Read the model definition and answer for the solid it produces. Units are mm, in the model's axes. Give positions to 0.01 mm unless a question says otherwise; leave off trailing zeros. Write each loop counter-clockwise with the first axis right and the second up, starting at its lowest first coordinate (ties: lowest second). Pieces come first, ordered by that corner, then holes. Notation, with made-up numbers: (50.25, 36) -> (66.25, 36) arc R26 cw to (66.25, 64) -> close; hole circle Ø5 at (-33, 80). An arc over 180 degrees is marked (long way). Write item = value, one per line.
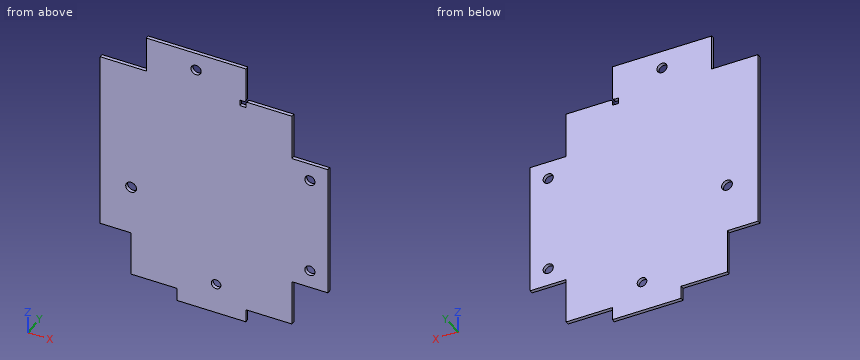
from build123d import *

# Parameters (mm, degrees)
CROQUIS1_W              = 190
CROQUIS1_H              = 230
SALIENTE_EXTRUIR2_DEPTH = 3
CROQUIS3_W              = 30
CROQUIS3_H              = 30
CORTAR_EXTRUIR1_DEPTH   = 10
CROQUIS5_W              = 38.5
CROQUIS5_H              = 30
CORTAR_EXTRUIR2_DEPTH   = 10
CROQUIS6_W              = 30
CROQUIS6_H              = 38.5
CORTAR_EXTRUIR3_DEPTH   = 10
CROQUIS7_W              = 38.5
CROQUIS7_H              = 30
CORTAR_EXTRUIR4_DEPTH   = 10
CORTAR_EXTRUIR12_DEPTH  = 10
CROQUIS11_W             = 5
CROQUIS11_H             = 5
CORTAR_EXTRUIR13_DEPTH  = 10
CORTAR_EXTRUIR14_DEPTH  = 10
CORTAR_EXTRUIR15_DEPTH  = 10
CORTAR_EXTRUIR16_DEPTH  = 10
CROQUIS15_W             = 30
CROQUIS15_H             = 38.5
CORTAR_EXTRUIR17_DEPTH  = 10
CROQUIS16_W             = 25.5
CROQUIS16_H             = 48.5
CORTAR_EXTRUIR18_DEPTH  = 10
CROQUIS17_W             = 24
CROQUIS17_H             = 11
CORTAR_EXTRUIR19_DEPTH  = 10
CROQUIS18_W             = 14.5
CROQUIS18_H             = 11
CORTAR_EXTRUIR20_DEPTH  = 10
CROQUIS19_R             = 4.25
CORTAR_EXTRUIR21_DEPTH  = 10
CROQUIS20_R             = 4.25
CORTAR_EXTRUIR22_DEPTH  = 10
CROQUIS21_R             = 4.5
CORTAR_EXTRUIR23_DEPTH  = 10
CROQUIS22_R             = 4
CORTAR_EXTRUIR24_DEPTH  = 10
CROQUIS23_W             = 30
CROQUIS23_H             = 38.5
CORTAR_EXTRUIR25_DEPTH  = 10
CROQUIS24_R             = 4.25
CORTAR_EXTRUIR26_DEPTH  = 10
SALIENTE_EXTRUIR4_DEPTH = 3
CROQUIS26_W             = 38.5
CROQUIS26_H             = 11
CORTAR_EXTRUIR27_DEPTH  = 30


with BuildPart() as part:
    # Croquis1 → Saliente-Extruir2 (new body)
    with BuildSketch(Plane(origin=(0, 0, 0), x_dir=(1, 0, 0), z_dir=(0, 1, 0))):
        Rectangle(CROQUIS1_W, CROQUIS1_H)
    extrude(amount=SALIENTE_EXTRUIR2_DEPTH)

    # Croquis3 → Cortar-Extruir1 (cut)
    with BuildSketch(Plane(origin=(0, 3, 0), x_dir=(1, 0, 0), z_dir=(0, 1, 0))):
        with Locations((80, -100)):
            Rectangle(CROQUIS3_W, CROQUIS3_H)
    extrude(amount=-CORTAR_EXTRUIR1_DEPTH, mode=Mode.SUBTRACT)

    # Croquis5 → Cortar-Extruir2 (cut)
    with BuildSketch(Plane(origin=(0, 3, 0), x_dir=(1, 0, 0), z_dir=(0, 1, 0))):
        with Locations((45.75, -100)):
            Rectangle(CROQUIS5_W, CROQUIS5_H)
    extrude(amount=-CORTAR_EXTRUIR2_DEPTH, mode=Mode.SUBTRACT)

    # Croquis6 → Cortar-Extruir3 (cut)
    with BuildSketch(Plane(origin=(0, 3, 0), x_dir=(1, 0, 0), z_dir=(0, 1, 0))):
        with Locations((80, -65.75)):
            Rectangle(CROQUIS6_W, CROQUIS6_H)
    extrude(amount=-CORTAR_EXTRUIR3_DEPTH, mode=Mode.SUBTRACT)

    # Croquis7 → Cortar-Extruir4 (cut)
    with BuildSketch(Plane(origin=(0, 3, 0), x_dir=(1, 0, 0), z_dir=(0, 1, 0))):
        with Locations((-75.75, -100)):
            Rectangle(CROQUIS7_W, CROQUIS7_H)
    extrude(amount=-CORTAR_EXTRUIR4_DEPTH, mode=Mode.SUBTRACT)

    # Croquis9 → Cortar-Extruir12 (cut)
    with BuildSketch(Plane(origin=(0, 3, 0), x_dir=(1, 0, 0), z_dir=(0, 1, 0))):
        Polygon((26.5, -85), (26.5, -85.75), (25.75, -85), (26.5, -84.25), (27.25, -85), align=None)
    extrude(amount=-CORTAR_EXTRUIR12_DEPTH, mode=Mode.SUBTRACT)

    # Croquis11 → Cortar-Extruir13 (cut)
    with BuildSketch(Plane(origin=(0, 3, 0), x_dir=(1, 0, 0), z_dir=(0, 1, 0))):
        with Locations((24, -82.5)):
            Rectangle(CROQUIS11_W, CROQUIS11_H)
    extrude(amount=-CORTAR_EXTRUIR13_DEPTH, mode=Mode.SUBTRACT)

    # Croquis12 → Cortar-Extruir14 (cut)
    with BuildSketch(Plane(origin=(0, 3, 0), x_dir=(1, 0, 0), z_dir=(0, 1, 0))):
        Polygon((26.5, -85.75), (25.75, -85), (25.573223305, -85.176776695), (26.323223305, -85.926776695), align=None)
    extrude(amount=-CORTAR_EXTRUIR14_DEPTH, mode=Mode.SUBTRACT)

    # Croquis13 → Cortar-Extruir15 (cut)
    with BuildSketch(Plane(origin=(0, 3, 0), x_dir=(1, 0, 0), z_dir=(0, 1, 0))):
        Polygon((26.5, -84.25), (27.25, -85), (27.426776695, -84.823223305), (26.676776695, -84.073223305), align=None)
    extrude(amount=-CORTAR_EXTRUIR15_DEPTH, mode=Mode.SUBTRACT)

    # Croquis14 → Cortar-Extruir16 (cut)
    with BuildSketch(Plane(origin=(0, 3, 0), x_dir=(1, 0, 0), z_dir=(0, 1, 0))):
        Polygon((25.573223305, -85.176776695), (25.75, -85), (25.002200766, -84.252200766), (24.82542407, -84.428977461), align=None)
        Polygon((26.323223305, -85.926776695), (26.5, -85.75), (26.914058622, -86.164058622), (26.737281927, -86.340835317), align=None)
        Polygon((27.426776695, -84.823223305), (27.25, -85), (27.599112283, -85.349112283), (27.775888978, -85.172335588), align=None)
        Polygon((26.676776695, -84.073223305), (26.5, -84.25), (26.076932461, -83.826932461), (26.253709156, -83.650155766), align=None)
    extrude(amount=-CORTAR_EXTRUIR16_DEPTH, mode=Mode.SUBTRACT)

    # Croquis15 → Cortar-Extruir17 (cut)
    with BuildSketch(Plane(origin=(0, 3, 0), x_dir=(1, 0, 0), z_dir=(0, 1, 0))):
        with Locations((80, 95.75)):
            Rectangle(CROQUIS15_W, CROQUIS15_H)
    extrude(amount=-CORTAR_EXTRUIR17_DEPTH, mode=Mode.SUBTRACT)

    # Croquis16 → Cortar-Extruir18 (cut)
    with BuildSketch(Plane(origin=(0, 3, 0), x_dir=(1, 0, 0), z_dir=(0, 1, 0))):
        with Locations((-82.25, 90.75)):
            Rectangle(CROQUIS16_W, CROQUIS16_H)
    extrude(amount=-CORTAR_EXTRUIR18_DEPTH, mode=Mode.SUBTRACT)

    # Croquis17 → Cortar-Extruir19 (cut)
    with BuildSketch(Plane(origin=(0, 3, 0), x_dir=(1, 0, 0), z_dir=(0, 1, 0))):
        with Locations((-57.5, 109.5)):
            Rectangle(CROQUIS17_W, CROQUIS17_H)
    extrude(amount=-CORTAR_EXTRUIR19_DEPTH, mode=Mode.SUBTRACT)

    # Croquis18 → Cortar-Extruir20 (cut)
    with BuildSketch(Plane(origin=(0, 3, 0), x_dir=(1, 0, 0), z_dir=(0, 1, 0))):
        with Locations((-38.25, 109.5)):
            Rectangle(CROQUIS18_W, CROQUIS18_H)
    extrude(amount=-CORTAR_EXTRUIR20_DEPTH, mode=Mode.SUBTRACT)

    # Croquis19 → Cortar-Extruir21 (cut)
    with BuildSketch(Plane(origin=(0, 3, 0), x_dir=(1, 0, 0), z_dir=(0, 1, 0))):
        with Locations(Location((80, 61.5, 0), (0, 0, 270))):
            Circle(CROQUIS19_R)
        with Locations(Location((80, -31.5, 0), (0, 0, 270))):
            Circle(CROQUIS19_R)
    extrude(amount=-CORTAR_EXTRUIR21_DEPTH, mode=Mode.SUBTRACT)

    # Croquis20 → Cortar-Extruir22 (cut)
    with BuildSketch(Plane(origin=(0, 3, 0), x_dir=(1, 0, 0), z_dir=(0, 1, 0))):
        with Locations(Location((-15, -100, 0), (0, 0, 270))):
            Circle(CROQUIS20_R)
    extrude(amount=-CORTAR_EXTRUIR22_DEPTH, mode=Mode.SUBTRACT)

    # Croquis21 → Cortar-Extruir23 (cut)
    with BuildSketch(Plane(origin=(0, 3, 0), x_dir=(1, 0, 0), z_dir=(0, 1, 0))):
        with Locations(Location((-69.25, 25, 0), (0, 0, 270))):
            Circle(CROQUIS21_R)
    extrude(amount=-CORTAR_EXTRUIR23_DEPTH, mode=Mode.SUBTRACT)

    # Croquis22 → Cortar-Extruir24 (cut)
    with BuildSketch(Plane(origin=(0, 3, 0), x_dir=(1, 0, 0), z_dir=(0, 1, 0))):
        with Locations(Location((1.7, 89.25, 0), (0, 0, 270))):
            Circle(CROQUIS22_R)
    extrude(amount=-CORTAR_EXTRUIR24_DEPTH, mode=Mode.SUBTRACT)

    # Croquis23 → Cortar-Extruir25 (cut)
    with BuildSketch(Plane(origin=(0, 3, 0), x_dir=(1, 0, 0), z_dir=(0, 1, 0))):
        with Locations((80, 84.75)):
            Rectangle(CROQUIS23_W, CROQUIS23_H)
    extrude(amount=-CORTAR_EXTRUIR25_DEPTH, mode=Mode.SUBTRACT)

    # Croquis24 → Cortar-Extruir26 (cut)
    with BuildSketch(Plane(origin=(0, 3, 0), x_dir=(1, 0, 0), z_dir=(0, 1, 0))):
        with Locations(Location((80, 50.5, 0), (0, 0, 270))):
            Circle(CROQUIS24_R)
    extrude(amount=-CORTAR_EXTRUIR26_DEPTH, mode=Mode.SUBTRACT)

    # Croquis25 → Saliente-Extruir4 (add)
    with BuildSketch(Plane(origin=(0, 3, 0), x_dir=(1, 0, 0), z_dir=(0, 1, 0))):
        with BuildLine():
            Line((78.563859338, 65.5), (81.436140662, 65.5))
            ThreePointArc((81.436140662, 65.5), (80, 57.25), (78.563859338, 65.5))
        make_face()
    extrude(amount=-SALIENTE_EXTRUIR4_DEPTH)

    # Croquis26 → Cortar-Extruir27 (cut)
    with BuildSketch(Plane(origin=(0, 3, 0), x_dir=(1, 0, 0), z_dir=(0, 1, 0))):
        with Locations((45.75, 109.5)):
            Rectangle(CROQUIS26_W, CROQUIS26_H)
    extrude(amount=-CORTAR_EXTRUIR27_DEPTH, mode=Mode.SUBTRACT)


solid = part.part
(1) Given P1, Ø0.9, axis at y = 1.5, z = -91.5, coming from the -X side; P2, Ø0.9, axis at x = 39, y = 1.5, coming from the +Z side; P3, Ø0.9, axis at x = -78.5, y = 2, coming from the -Z side; P4, Ø6, axis at x = 30, z = -63, coming from the -Y side, each flat-ended and moving along its own axis, determine where each tip first touches the part or whether it passes through.
Checks:
P1 = -69.5
P2 = 85
P3 = -66.5
P4 = 0
(2) The part is cut by section A-A on x = -15. Determine the outline of the cut face in (y, z).
Checks:
outline = (0, -115) -> (3, -115) -> (3, 95.75) -> (0, 95.75) -> close; (0, 104.25) -> (3, 104.25) -> (3, 115) -> (0, 115) -> close
(3) The part is cut by section D-D on x = 80. Determine the outline of the cut face in (y, z).
Checks:
outline = (0, -65.5) -> (3, -65.5) -> (3, -54.75) -> (0, -54.75) -> close; (0, -46.25) -> (3, -46.25) -> (3, 27.25) -> (0, 27.25) -> close; (0, 35.75) -> (3, 35.75) -> (3, 46.5) -> (0, 46.5) -> close
(4) Consider L1, parallel to X at y = 0.95, z = -50.5; L2, parallel to X at y = 0.75, z = 100.5; L3, parallel to Z at x = -51, y = 2.2. Determine where each line is inside the solid, lowest interval first.
Checks:
L1 = -95 to 75.75, 84.25 to 95
L2 = -56.5 to -19.22, -10.78 to 26.5
L3 = -104 to 115
(5) The part is cut by section C-C on y = 0.75. Count the separate pieces of the cut face and the enclosed holes in it, plus the area to 3 significant figures.
Checks:
separate_pieces = 1
enclosed_holes = 5
area = 35,500 mm²
(6) The part is cut by section B-B on z = -25. Determine the outline of the cut face in (x, y), plus the area to 3 significant figures.
Checks:
outline = (-95, 0) -> (-73.75, 0) -> (-73.75, 3) -> (-95, 3) -> close; (-64.75, 0) -> (95, 0) -> (95, 3) -> (-64.75, 3) -> close
area = 543 mm²
